from build123d import *

# Parameters (mm, degrees)
SZKIC1_R                    = 1
SZKIC1_R_2                  = 3
DODANIE_WYCI_GNI_CIE1_DEPTH = 5
SZKIC1_3_R                  = 10.570763761
SZKIC1_3_R_2                = 3
SZKIC1_3_R_3                = 1
DODANIE_WYCI_GNI_CIE2_DEPTH = 10
SZKIC1_4_R                  = 3
DODANIE_WYCI_GNI_CIE3_DEPTH = 50


with BuildPart() as part:
    # Szkic1 → Dodanie-wyci_gni_cie1 (new body)
    with BuildSketch(Plane.XY):
        with BuildLine():
            Line((-50.67287635, 5.055665151), (-9.235111676, 10.570763761))
            ThreePointArc((-9.235111676, 10.570763761), (0, 11.182632843), (9.235111676, 10.570763761))
            Line((9.235111676, 10.570763761), (50.67287635, 5.055665151))
            ThreePointArc((50.67287635, 5.055665151), (55.100246338, 0), (50.67287635, -5.055665151))
            Line((50.67287635, -5.055665151), (9.235111676, -10.570763761))
            ThreePointArc((9.235111676, -10.570763761), (0, -11.182632843), (-9.235111676, -10.570763761))
            Line((-9.235111676, -10.570763761), (-50.67287635, -5.055665151))
            ThreePointArc((-50.67287635, -5.055665151), (-55.100246338, 0), (-50.67287635, 5.055665151))
        make_face()
        with Locations((-5.656854249, 5.656854249)):
            Circle(SZKIC1_R, mode=Mode.SUBTRACT)
        with Locations((-8, 0)):
            Circle(SZKIC1_R, mode=Mode.SUBTRACT)
        with Locations((0, 8)):
            Circle(SZKIC1_R, mode=Mode.SUBTRACT)
        with Locations((5.656854249, 5.656854249)):
            Circle(SZKIC1_R, mode=Mode.SUBTRACT)
        with Locations((-50, 0)):
            Circle(SZKIC1_R_2, mode=Mode.SUBTRACT)
        with Locations((50, 0)):
            Circle(SZKIC1_R_2, mode=Mode.SUBTRACT)
        with Locations((8, 0)):
            Circle(SZKIC1_R, mode=Mode.SUBTRACT)
        with Locations((5.656854249, -5.656854249)):
            Circle(SZKIC1_R, mode=Mode.SUBTRACT)
        with Locations((0, -8)):
            Circle(SZKIC1_R, mode=Mode.SUBTRACT)
        with Locations((-5.656854249, -5.656854249)):
            Circle(SZKIC1_R, mode=Mode.SUBTRACT)
    extrude(amount=DODANIE_WYCI_GNI_CIE1_DEPTH)

    # Szkic1_3 → Dodanie-wyci_gni_cie2 (add)
    with BuildSketch(Plane.XY):
        Circle(SZKIC1_3_R)
        Circle(SZKIC1_3_R_2, mode=Mode.SUBTRACT)
        with Locations((-5.656854249, 5.656854249)):
            Circle(SZKIC1_3_R_3, mode=Mode.SUBTRACT)
        with Locations((-8, 0)):
            Circle(SZKIC1_3_R_3, mode=Mode.SUBTRACT)
        with Locations((0, 8)):
            Circle(SZKIC1_3_R_3, mode=Mode.SUBTRACT)
        with Locations((5.656854249, 5.656854249)):
            Circle(SZKIC1_3_R_3, mode=Mode.SUBTRACT)
        with Locations((8, 0)):
            Circle(SZKIC1_3_R_3, mode=Mode.SUBTRACT)
        with Locations((5.656854249, -5.656854249)):
            Circle(SZKIC1_3_R_3, mode=Mode.SUBTRACT)
        with Locations((0, -8)):
            Circle(SZKIC1_3_R_3, mode=Mode.SUBTRACT)
        with Locations((-5.656854249, -5.656854249)):
            Circle(SZKIC1_3_R_3, mode=Mode.SUBTRACT)
    extrude(amount=DODANIE_WYCI_GNI_CIE2_DEPTH)

    # Szkic1_4 → Dodanie-wyci_gni_cie3 (add)
    with BuildSketch(Plane.XY):
        Circle(SZKIC1_4_R)
    extrude(amount=DODANIE_WYCI_GNI_CIE3_DEPTH)


solid = part.part
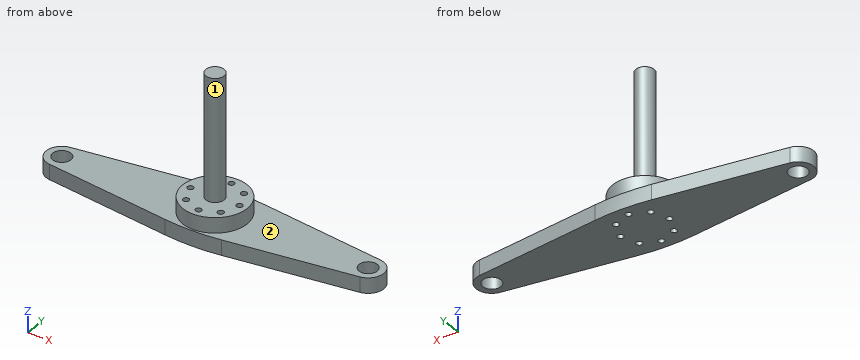
The listing builds one solid part. Answer for the finished solid, in the listing's coordinates (mm). Face numbers are marked on the shaded views. Coordinates: 2 decimals unless noted, no trailing zeros. Write each loop counter-clockwise with the first axis right and the second up, starting at its lowest first coordinate (ties: lowest second). Pieces come first, ordered by that corner, then holes. Notation, with made-up numbers: (-27.5, 60) - (-19.5, 60) arc R31 cw to (-19.5, 89) - close; hole circle Ø9 at (39.5, -10.5). An arc over 180 degrees is marked (long way). Put each result on its own line as item: value.
1. The part is cut by section C-C on z = 17.5. Give the vertices of the cut face in (x, y).
Answer sheet:
outline: circle Ø6 at (0, 0)
2. Determine the mould class of the marked faces 1 and 2 for opening direction X: pulls with the +X half, pulls with the -X half, needs draft (parallel to the pull), parting line crosses it, or undercut.
Answer sheet:
face 1: parting line crosses it
face 2: needs draft
3. The part is cut by section B-B on x = 0. Give the vertices of the cut face in (y, z).
Answer sheet:
outline: (-11.18, 0) - (-9, 0) - (-9, 10) - (-10.57, 10) - (-10.57, 5) - (-11.18, 5) - close; (-7, 0) - (7, 0) - (7, 10) - (3, 10) - (3, 50) - (-3, 50) - (-3, 10) - (-7, 10) - close; (9, 0) - (11.18, 0) - (11.18, 5) - (10.57, 5) - (10.57, 10) - (9, 10) - close
4. The part is cut by section A-A on y = -8. Give the vertices of the cut face in (x, z).
Answer sheet:
outline: (-28.55, 0) - (-1, 0) - (-1, 10) - (-6.91, 10) - (-6.91, 5) - (-28.55, 5) - close; (1, 0) - (28.55, 0) - (28.55, 5) - (6.91, 5) - (6.91, 10) - (1, 10) - close
5. Find the intervals of material crossed by line 1 along Z through (x, y) = (9, 6.5); line 2 along Z through (x, y) = (9, -0.5); line 3 along Y through (x, z) = (-8, 3.25), in increasing order. Write a range as from..to.
Answer sheet:
line 1: z = 0..5
line 2: z = 0..10
line 3: y = -10.72..-1, 1..10.72
6. Flat-ended cylindrical pins translate along their axes: pin 1 Ø4 at (x, y) = (11.5, 7.5) entering from -Z; pin 2 Ø6 at (x, y) = (34, 2.5) entering from +Z; pin 3 Ø2.5 at (x, y) = (-5.66, 5.66) entering from +Z; pin 4 Ø10 at (x, z) = (31, 7.5) entering from +Y. Find the tip coordinate at first contact, or state that the pin passes through.
Answer sheet:
pin 1: stops at z = 0
pin 2: stops at z = 5
pin 3: stops at z = 10
pin 4: stops at y = 8.25
7. The part is cut by section D-D on x = 46. Give the vertices of the cut face in (y, z), plus the area to 3 significant figures.
Answer sheet:
outline: (-5.68, 0) - (5.68, 0) - (5.68, 5) - (-5.68, 5) - close
area: 56.8 mm^2
